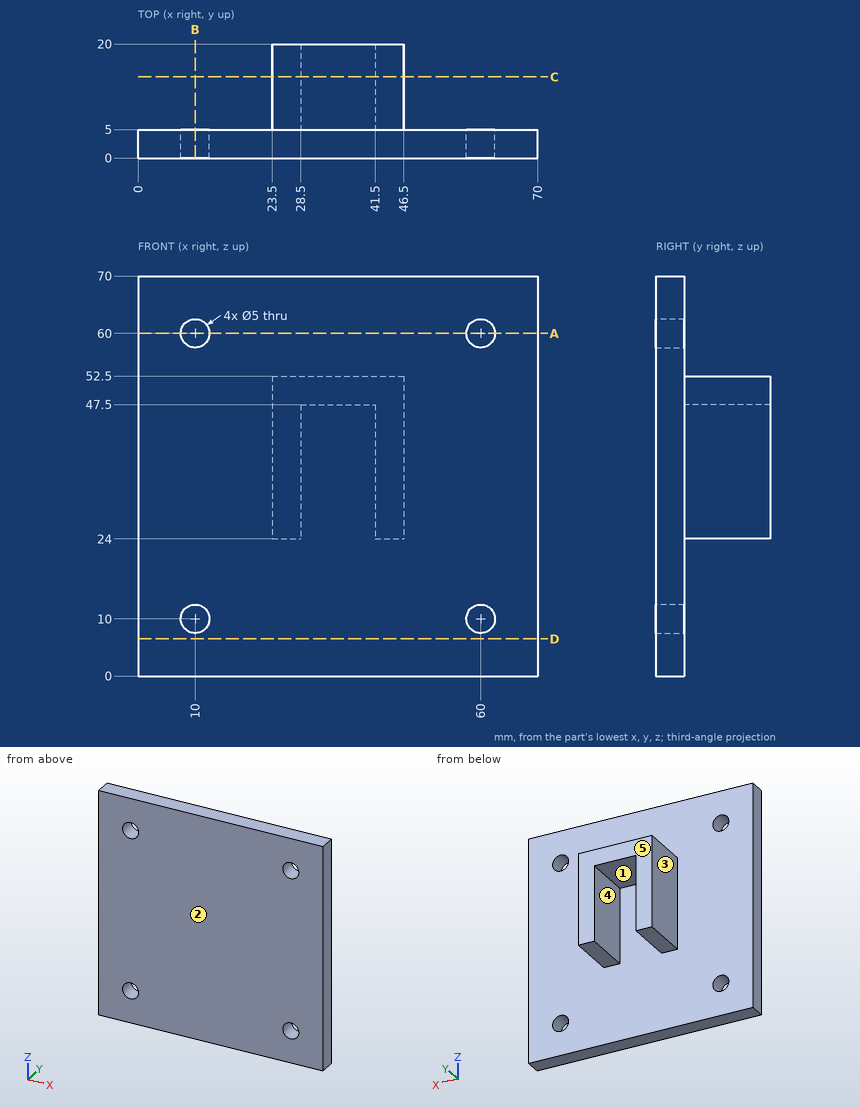
Geometry: see drawing. Coordinates: mm, zero at the bounding-box minimum. A direction names the side the tool comes from. Give positions to 0.01 mm unless a question says otherwise; leave off trailing zeros. Write each loop counter-clockwise with the first axis right and the second up, starting at its lowest first coordinate (ties: lowest second). Pieces come first, ordered by that corner, then holes. Notation, with made-up numbers: (78, 26.5) - (102, 26.5) arc R15 ccw to (102, 37.5) - close; hole circle Ø7 at (44, 39.25). An arc over 180 degrees is marked (long way). Return JSON: item names as keys, results as strings. Group by question number.
1) Section C-C on y = 14.25. Return the cut outline in (x, z), plus the area to 3 significant figures.
2) Set-up query: the marked faces 4 and 5. Return all of +Z, -Z, +X, -X, +Y, -Y with unobstructed straight access to the full face (end or side cutting, diameter ignored); none if empty.
3) Section B-B on x = 10. Return the cut outline in (y, z), plus the area to 3 significant figures.
4) Section D-D on z = 6.5. Return the cut outline in (x, y), plus the area to 3 significant figures.
5) First-contact query: P1, Ø3, axis at x = 32.5, z = 41.5, coming from the +Y side; P2, Ø12, axis at y = 14, z = 36, coming from the +X side; P3, Ø12, axis at x = 34.5, y = 14, coming from the +Z side; P4, Ø4, axis at x = 60, z = 60, coming from the -Y side. Flat tips, straight axial feed; report the tip coordinate or a pass-through.
6) Line query: line 1 (X direction, y = 1.75, z = 10); line 2 (X direction, y = 18, z = 40); line 3 (Y direction, x = 33, z = 16.5). Output: solid intervals per line, ascending.
7) Section A-A on z = 60. Return the cut outline in (x, y).
8) Mould query, pull axis X, two halves, no side actions, for the marked faces 1, 2 and 3. Classes: released by +X, released by -X, zero draft, split by the parting line, or undercut.
Filled in:
{
 "1": {"outline": "(23.5, 24) - (28.5, 24) - (28.5, 47.5) - (41.5, 47.5) - (41.5, 24) - (46.5, 24) - (46.5, 52.5) - (23.5, 52.5) - close", "area": "350 mm^2"},
 "2": {"face 4": "-Z, +Y", "face 5": "+Z, -Z, +X, -X, +Y"},
 "3": {"outline": "(0, 0) - (5, 0) - (5, 7.5) - (0, 7.5) - close; (0, 12.5) - (5, 12.5) - (5, 57.5) - (0, 57.5) - close; (0, 62.5) - (5, 62.5) - (5, 70) - (0, 70) - close", "area": "300 mm^2"},
 "4": {"outline": "(0, 0) - (70, 0) - (70, 5) - (0, 5) - close", "area": "350 mm^2"},
 "5": {"P1": "stops at y = 5", "P2": "stops at x = 46.5", "P3": "stops at z = 52.5", "P4": "passes through"},
 "6": {"line 1": "x = 0 to 7.5, 12.5 to 57.5, 62.5 to 70", "line 2": "x = 23.5 to 28.5, 41.5 to 46.5", "line 3": "y = 0 to 5"},
 "7": {"outline": "(0, 0) - (7.5, 0) - (7.5, 5) - (0, 5) - close; (12.5, 0) - (57.5, 0) - (57.5, 5) - (12.5, 5) - close; (62.5, 0) - (70, 0) - (70, 5) - (62.5, 5) - close"},
 "8": {"face 1": "undercut", "face 2": "zero draft", "face 3": "released by -X"}
}
